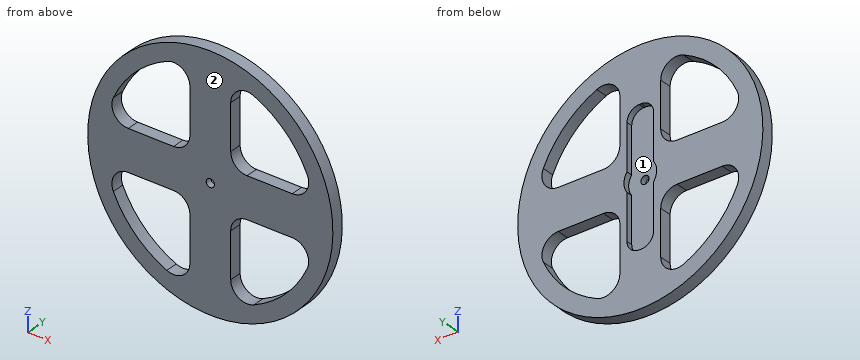
from build123d import *

# Parameters (mm, degrees)
SKETCH1_R           = 30
BOSS_EXTRUDE1_DEPTH = 3
CUT_EXTRUDE1_DEPTH  = 1.5
CUT_EXTRUDE2_DEPTH  = 3
SKETCH4_R           = 1
CUT_EXTRUDE3_DEPTH  = 3
FILLET1_R           = 4
FILLET2_R           = 3


with BuildPart() as part:
    # Sketch1 → Boss-Extrude1 (new body)
    with BuildSketch(Plane(origin=(0, 0, 0), x_dir=(1, 0, 0), z_dir=(0, 1, 0))):
        with Locations(Location((0, 0, 0), (0, 0, 270))):
            Circle(SKETCH1_R)
    extrude(amount=BOSS_EXTRUDE1_DEPTH)

    # Sketch2 → Cut-Extrude1 (cut)
    with BuildSketch(Plane(origin=(0, 3, 0), x_dir=(1, 0, 0), z_dir=(0, 1, 0))):
        with BuildLine():
            Line((-3.25, 16.5), (-3.25, 2.331844763))
            ThreePointArc((-3.25, 2.331844763), (-4, 0), (-3.25, -2.331844763))
            Line((-3.25, -2.331844763), (-3.25, -16.5))
            Line((-3.25, -16.5), (3.25, -16.5))
            Line((3.25, -16.5), (3.25, -2.331844763))
            ThreePointArc((3.25, -2.331844763), (4, 0), (3.25, 2.331844763))
            Line((3.25, 2.331844763), (3.25, 16.5))
            Line((3.25, 16.5), (-3.25, 16.5))
        make_face()
    extrude(amount=-CUT_EXTRUDE1_DEPTH, mode=Mode.SUBTRACT)

    # Sketch3 → Cut-Extrude2 (cut)
    with BuildSketch(Plane(origin=(0, 3, 0), x_dir=(1, 0, 0), z_dir=(0, 1, 0))):
        with BuildLine():
            Line((-5, -25.514701644), (-5, -5))
            Line((-5, -5), (-25.514701644, -5))
            ThreePointArc((-25.514701644, -5), (-18.384776311, -18.384776311), (-5, -25.514701644))
        make_face()
        with BuildLine():
            Line((5, -25.514701644), (5, -5))
            Line((5, -5), (25.514701644, -5))
            ThreePointArc((25.514701644, -5), (18.384776311, -18.384776311), (5, -25.514701644))
        make_face()
        with BuildLine():
            Line((25.514701644, 5), (5, 5))
            Line((5, 5), (5, 25.514701644))
            ThreePointArc((5, 25.514701644), (18.384776311, 18.384776311), (25.514701644, 5))
        make_face()
        with BuildLine():
            Line((-5, 5), (-5, 25.514701644))
            ThreePointArc((-5, 25.514701644), (-18.384776311, 18.384776311), (-25.514701644, 5))
            Line((-25.514701644, 5), (-5, 5))
        make_face()
    extrude(amount=-CUT_EXTRUDE2_DEPTH, mode=Mode.SUBTRACT)

    # Sketch4 → Cut-Extrude3 (cut)
    with BuildSketch(Plane.XZ):
        with Locations(Location((0, 0, 0), (0, 0, 270))):
            Circle(SKETCH4_R)
    extrude(amount=-CUT_EXTRUDE3_DEPTH, mode=Mode.SUBTRACT)

    # Fillet1
    fillet1_edges = [part.edges().sort_by_distance(p)[0] for p in [
        (-25.514701644, 1.5, -5),
        (-5, 1.5, -25.514701644),
        (-5, 1.5, -5),
        (25.514701644, 1.5, 5),
        (5, 1.5, 25.514701644),
        (5, 1.5, 5),
        (5, 1.5, -25.514701644),
        (25.514701644, 1.5, -5),
        (5, 1.5, -5),
        (-5, 1.5, 25.514701644),
        (-25.514701644, 1.5, 5),
        (-5, 1.5, 5),
    ]]
    fillet(fillet1_edges, radius=FILLET1_R)

    # Fillet2
    fillet2_edges = [part.edges().sort_by_distance(p)[0] for p in [
        (3.25, 2.25, 16.5),
        (-3.25, 2.25, 16.5),
        (-3.25, 2.25, -16.5),
        (3.25, 2.25, -16.5),
    ]]
    fillet(fillet2_edges, radius=FILLET2_R)


solid = part.part
Input: part model. Units: mm. Frame: model coordinates. Face numbers are marked on the shaded views. Round coordinates to 2 decimals unless told otherwise and drop trailing zeros. Write each loop counter-clockwise with the first axis right and the second up, starting at its lowest first coordinate (ties: lowest second). Pieces come first, ordered by that corner, then holes.
1) Cut plane B-B (z = 0). Return the cut outline in (x, y), then the cut area to 3 significant figures.
2) Cut plane D-D (z = 6). Return the cut outline in (x, y), then the cut area to 3 significant figures.
3) Draft query along X for the marked faces 1 and 2. Return one class per face: pulls with the +X half, pulls with the -X half, needs draft (parallel to the pull), parting line crosses it, or undercut.
4) Contact query for flat-ended pins moving along their axis: P1, Ø6.5, axis at x = 1.5, z = 8, coming from the +Y side; P2, Ø2.5, axis at x = 0, z = 0, coming from the +Y side; P3, Ø0.9, axis at x = -13.5, y = 1, coming from the -Z side; P4, Ø1.5, axis at y = 1, z = 13, coming from the +X side (3 decimals). Output: stop coordinate, or through.
5) Cut plane A-A (y = 1). Return the cut outline in (x, z).
6) Cut plane C-C (x = -8). Return the cut outline in (y, z), then the cut area to 3 significant figures.
7) Ray query, L1, parallel to X at y = 0.35, z = 0; L2, parallel to X at y = 1.15, z = -21; L3, parallel to X at y = 0.1, z = 22. Return the intervals inside material, ascending.
Geometry says:
1. outline: (-30, 0) - (-1, 0) - (-1, 1.5) - (-4, 1.5) - (-4, 3) - (-30, 3) - close; (1, 0) - (30, 0) - (30, 3) - (4, 3) - (4, 1.5) - (1, 1.5) - close
1. area: 165 mm2
2. outline: (-29.39, 0) - (-22.72, 0) - (-22.72, 3) - (-29.39, 3) - close; (-6.35, 0) - (6.35, 0) - (6.35, 3) - (3.25, 3) - (3.25, 1.5) - (-3.25, 1.5) - (-3.25, 3) - (-6.35, 3) - close; (22.72, 0) - (29.39, 0) - (29.39, 3) - (22.72, 3) - close
2. area: 68.4 mm2
3. face 1: undercut
3. face 2: needs draft
4. P1: stops at y = 3
4. P2: stops at y = 1.5
4. P3: stops at z = -27.01
4. P4: stops at x = 27.385
5. outline: circle Ø60 at (0, 0); hole (-23.72, -10.64) arc R26 ccw to (-10.64, -23.72) arc R4 ccw to (-5, -20.07) - (-5, -9) arc R4 ccw to (-9, -5) - (-20.07, -5) arc R4 ccw to start; hole (-23.72, 10.64) arc R4 ccw to (-20.07, 5) - (-9, 5) arc R4 ccw to (-5, 9) - (-5, 20.07) arc R4 ccw to (-10.64, 23.72) arc R26 ccw to start; hole circle Ø2 at (0, 0); hole (5, -20.07) arc R4 ccw to (10.64, -23.72) arc R26 ccw to (23.72, -10.64) arc R4 ccw to (20.07, -5) - (9, -5) arc R4 ccw to (5, -9) - close; hole (5, 9) arc R4 ccw to (9, 5) - (20.07, 5) arc R4 ccw to (23.72, 10.64) arc R26 ccw to (10.64, 23.72) arc R4 ccw to (5, 20.07) - close
6. outline: (0, -28.91) - (3, -28.91) - (3, -23.95) - (0, -23.95) - close; (0, -5.13) - (3, -5.13) - (3, 5.13) - (0, 5.13) - close; (0, 23.95) - (3, 23.95) - (3, 28.91) - (0, 28.91) - close
6. area: 60.6 mm2
7. L1: x = -30 to -1, 1 to 30
7. L2: x = -21.42 to -15.33, -5.11 to 5.11, 15.33 to 21.42
7. L3: x = -20.4 to -13.86, -5.49 to 5.49, 13.86 to 20.4
